from build123d import *

# Parameters (mm, degrees)
SKETCH162_R      = 16.278821
EXTRUDE144_DEPTH = 4
ARRAY_X_COUNT    = 3
ARRAY_X_PITCH    = 55
ARRAY_Y_COUNT    = 2
ARRAY_Y_PITCH    = 55
EXTRUDE129_DEPTH = 2


with BuildPart() as array:
    # Sketch162 → Extrude144 (new body)
    with BuildSketch(Plane(origin=(0, 0, -37), x_dir=(1, 0, 0), z_dir=(0, 0, -1))):
        with Locations((222, -214.650925)):
            Circle(SKETCH162_R)
    extrude(amount=-EXTRUDE144_DEPTH)

    # Array X: Array ×3


with BuildPart() as array_1:
    add(array.part)
    with Locations(*[(i * ARRAY_X_PITCH, 0, 0) for i in range(1, ARRAY_X_COUNT)]):
        add(array.part)

    # Array Y: Array ×2


with BuildPart() as array_2:
    add(array_1.part)
    with Locations(*[(0, i * ARRAY_Y_PITCH, 0) for i in range(1, ARRAY_Y_COUNT)]):
        add(array_1.part)


with BuildPart() as cut009:
    # Sketch141 → Extrude129 (new body)
    with BuildSketch(Plane(origin=(0, 0, -34), x_dir=(1, 0, 0), z_dir=(0, 0, -1))):
        Polygon((215, -170), (205, -170), (195, -180), (191, -180), (191, -307), (268, -307), (268, -305.5), (292, -305.5), (292, -307), (365, -307), (365, -180), (347, -180), (337, -170), (327, -170), (327, -180), (215, -180), align=None)
    extrude(amount=EXTRUDE129_DEPTH)

    # Cut009: cut Array
    add(array_2.part, mode=Mode.SUBTRACT)


solid = cut009.part
Can you work these out from the model? Positions are in its coordinate system, mm. Coordinates: 2 decimals unless noted, no trailing zeros. Loops run counter-clockwise (first coordinate to the right, second up) from the corner with the lowest first, then second, coordinate; pieces in that order, holes last. Notation, with made-up numbers: (45, 65) - (55, 65) arc R10 ccw to (55, 81) - close; hole circle Ø9 at (59, 35.25). An arc over 180 degrees is marked (long way). Answer as a JSON object with one key per item and string values. Group by question number.
Item 1: If we section it at D-D (x = 249.5): List the corners of the cut face in (y, z) for me.
Item 2: If we section it at B-B (y = 273.5): List the corners of the cut face in (x, z) for me, plus the area to 3 significant figures.
Item 3: If we section it at A-A (x = 277): List the corners of the cut face in (y, z) for me.
Item 4: If we section it at C-C (x = 332): List the corners of the cut face in (y, z) for me.
Item 5: For pin 1 (0.6 mm diameter, centred on x = 194, z = -35, fed in from -Y); pin 2 (0.6 mm diameter, centred on y = 177.5, z = -35.5, fed in from +X); pin 3 (0.6 mm diameter, centred on y = 176, z = -35, fed in from -X), each with a flat end and sliding along its axis, tell me the tip position at first contact or that it passes through.
Item 6: If I drill on L1, parallel to Y at x = 222, z = -34.95; L2, parallel to Y at x = 332, z = -34.9; L3, parallel to X at y = 266, z = -34.4, over which ranges is the centre line in solid material (lowest first)? Write a range as from..to.
Item 7: If we mould it in two halves opening along X, with no side actions, what happens to faces 1 (the face through (200, 175, -35)), 2 (the face through (260.737, 213.935, -35.014)), 3 (the face through (342, 175, -35)), 4 (the face through (277, 238, -36))? For each: released by +X, released by -X, zero draft, split by the parting line, or undercut.
Returned:
{
 "1": {"outline": "(180, -36) - (307, -36) - (307, -34) - (180, -34) - close"},
 "2": {"outline": "(191, -36) - (206.18, -36) - (206.18, -34) - (191, -34) - close; (237.82, -36) - (261.18, -36) - (261.18, -34) - (237.82, -34) - close; (292.82, -36) - (316.18, -36) - (316.18, -34) - (292.82, -34) - close; (347.82, -36) - (365, -36) - (365, -34) - (347.82, -34) - close", "area": "158 mm²"},
 "3": {"outline": "(180, -36) - (198.37, -36) - (198.37, -34) - (180, -34) - close; (230.93, -36) - (253.37, -36) - (253.37, -34) - (230.93, -34) - close; (285.93, -36) - (305.5, -36) - (305.5, -34) - (285.93, -34) - close"},
 "4": {"outline": "(170, -36) - (198.37, -36) - (198.37, -34) - (170, -34) - close; (230.93, -36) - (253.37, -36) - (253.37, -34) - (230.93, -34) - close; (285.93, -36) - (307, -36) - (307, -34) - (285.93, -34) - close"},
 "5": {"pin 1": "stops at y = 180", "pin 2": "stops at x = 344.8", "pin 3": "stops at x = 198.7"},
 "6": {"L1": "y = 180..198.37, 230.93..253.37, 285.93..307", "L2": "y = 170..198.37, 230.93..253.37, 285.93..307", "L3": "x = 191..206.14, 237.86..261.14, 292.86..316.14, 347.86..365"},
 "7": {"face 1": "released by -X", "face 2": "undercut", "face 3": "released by +X", "face 4": "zero draft"}
}
